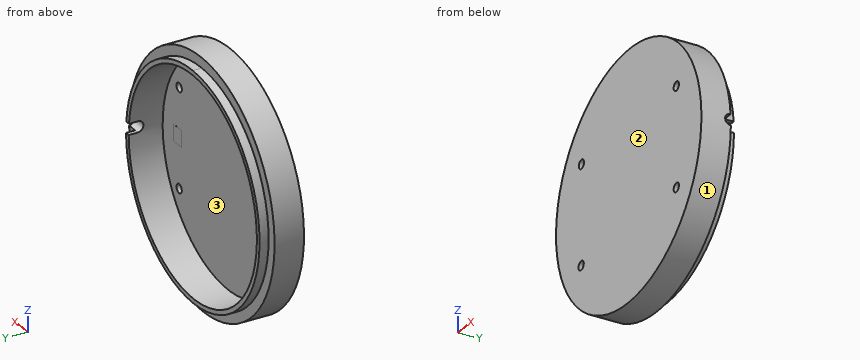
```python
from build123d import *

# Parameters (mm, degrees)
SKETCH2_R                = 55
BOSS_EXTRUDE2_DEPTH      = 13
SKETCH7_R                = 50.5
BOSS_EXTRUDE3_DEPTH      = 4
SKETCH8_R                = 48.5
CUT_EXTRUDE3_DEPTH       = 15
SKETCH9_R                = 2
SKETCH9_W                = 3.162660916
SKETCH9_H                = 2.60493009
CUT_EXTRUDE4_DEPTH       = 15
CUT_EXTRUDE5_DEPTH       = 20
CUT_EXTRUDE5_DEPTH_BACK  = 1
SKETCH10_R               = 2.5
BOSS_EXTRUDE5_DEPTH      = 0.01
BOSS_EXTRUDE5_DEPTH_BACK = 2
SKETCH11_W               = 6.274273212
SKETCH11_H               = 7.379534018
CUT_EXTRUDE6_REACH       = 81.618
CUT_EXTRUDE6_END_RADIUS  = 50.5
SKETCH13_W               = 5
SKETCH13_H               = 6.11505402


with BuildPart() as part:
    # Sketch2 → Boss-Extrude2 (new body)
    with BuildSketch(Plane(origin=(0, 0, 0), x_dir=(1, 0, 0), z_dir=(0, 1, 0))):
        with Locations(Location((0, 0, 0), (0, 0, 90))):
            Circle(SKETCH2_R)
    extrude(amount=BOSS_EXTRUDE2_DEPTH)

    # Sketch7 → Boss-Extrude3 (add)
    with BuildSketch(Plane(origin=(0, 13, 0), x_dir=(1, 0, 0), z_dir=(0, 1, 0))):
        with Locations(Location((0, 0, 0), (0, 0, 270))):
            Circle(SKETCH7_R)
    extrude(amount=BOSS_EXTRUDE3_DEPTH)

    # Sketch8 → Cut-Extrude3 (cut)
    with BuildSketch(Plane(origin=(0, 17, 0), x_dir=(1, 0, 0), z_dir=(0, 1, 0))):
        with Locations(Location((0, 0, 0), (0, 0, 270))):
            Circle(SKETCH8_R)
    extrude(amount=-CUT_EXTRUDE3_DEPTH, mode=Mode.SUBTRACT)

    # Sketch9 → Cut-Extrude4 (cut)
    with BuildSketch(Plane(origin=(0, 2, 0), x_dir=(1, 0, 0), z_dir=(0, 1, 0))):
        with Locations(Location((36, -22, 0), (0, 0, 270))):
            Circle(SKETCH9_R)
        with Locations(Location((-36, 22, 0), (0, 0, 270))):
            Circle(SKETCH9_R)
        with Locations(Location((-35.8, -22, 0), (0, 0, 270))):
            Circle(SKETCH9_R)
        with Locations(Location((36, 22, 0), (0, 0, 270))):
            Circle(SKETCH9_R)
        with Locations((37.581330458, -0.802465045)):
            Rectangle(SKETCH9_W, SKETCH9_H)
    extrude(amount=-CUT_EXTRUDE4_DEPTH, mode=Mode.SUBTRACT)

    # Sketch10 → Cut-Extrude5 (cut, two sides: drawn at the far end of the back side and taken through both)
    with BuildSketch(Plane(origin=(36, 0, 0), x_dir=(0, 0, -1), z_dir=(1, 0, 0)).offset(-CUT_EXTRUDE5_DEPTH_BACK)):
        with Locations(Location((-2, 13, 0), (0, 0, 180))):
            Circle(SKETCH10_R)
    extrude(amount=CUT_EXTRUDE5_DEPTH + CUT_EXTRUDE5_DEPTH_BACK, mode=Mode.SUBTRACT)

    # Sketch11 → Boss-Extrude5 (add, two sides: drawn at the far end of the back side and taken through both)
    with BuildSketch(Plane(origin=(0, 2, 0), x_dir=(1, 0, 0), z_dir=(0, 1, 0)).offset(-BOSS_EXTRUDE5_DEPTH_BACK)):
        with Locations((37.193701051, -0.388212482)):
            Rectangle(SKETCH11_W, SKETCH11_H)
    extrude(amount=BOSS_EXTRUDE5_DEPTH + BOSS_EXTRUDE5_DEPTH_BACK)

    # Cut-Extrude6: up to this cylinder (the profile starts inside it)
    cut_extrude6_end = Plane(origin=(0, 16.057527, 0), z_dir=(0, -1, 0)) * Cylinder(CUT_EXTRUDE6_END_RADIUS, 265.236, mode=Mode.PRIVATE)
    # Sketch13 → Cut-Extrude6 (cut, up to the surface)
    with BuildSketch(Plane(origin=(0, 0, 0), x_dir=(0, 0, -1), z_dir=(1, 0, 0)), mode=Mode.PRIVATE) as cut_extrude6_sk1:
        with Locations((-2, 16.05752701)):
            Rectangle(SKETCH13_W, SKETCH13_H)
    cut_extrude6_tool1 = extrude(cut_extrude6_sk1.sketch, amount=CUT_EXTRUDE6_REACH, mode=Mode.PRIVATE) & cut_extrude6_end
    add(cut_extrude6_tool1.solids().sort_by_distance((0, 16.057527, 2))[0], mode=Mode.SUBTRACT)


solid = part.part
```
Input: part model. Units: mm. Frame: model coordinates. Face numbers are marked on the shaded views. Round coordinates to 2 decimals unless told otherwise and drop trailing zeros. Loops run counter-clockwise (first coordinate to the right, second up) from the corner with the lowest first, then second, coordinate; pieces in that order, holes last. Notation, with made-up numbers: (48.25, 21.25) -> (57.25, 21.25) arc R27 ccw to (57.25, 43.25) -> close; hole circle Ø4 at (6.25, -10). An arc over 180 degrees is marked (long way). Write each question's results on one line, items separated by ' | '.
1. Section B-B (x = 14.5). Return loops of the section in (y, z).
Geometry results:
outline: (0, -53.05) -> (13, -53.05) -> (13, -48.37) -> (17, -48.37) -> (17, -46.28) -> (2, -46.28) -> (2, 46.28) -> (17, 46.28) -> (17, 48.37) -> (13, 48.37) -> (13, 53.05) -> (0, 53.05) -> close
2. First-contact query: P1, Ø10, axis at y = 3.5, z = 24.5, coming from the +X side; P2, Ø5, axis at x = -41.5, y = 13, coming from the +Z side; P3, Ø10, axis at y = 2.5, z = 14.5, coming from the -X side. Flat tips, straight axial feed; report the tip coordinate or a pass-through.
Geometry results:
P1: x = 51.43 | P2: z = 38.78 | P3: x = -54.17
3. Section A-A (z = 22). Return loops of the section in (x, y).
Geometry results:
outline: (-50.41, 0) -> (-37.8, 0) -> (-37.8, 2) -> (-43.22, 2) -> (-43.22, 17) -> (-45.46, 17) -> (-45.46, 13) -> (-50.41, 13) -> close; (-33.8, 0) -> (34, 0) -> (34, 2) -> (-33.8, 2) -> close; (38, 0) -> (50.41, 0) -> (50.41, 13) -> (45.46, 13) -> (45.46, 17) -> (43.22, 17) -> (43.22, 2) -> (38, 2) -> close
4. Ray query, line 1 (X direction, y = 9.5, z = 0); line 2 (X direction, y = 0.45, z = 22); line 3 (X direction, y = 0.5, z = -22). Return the intervals inside material, ascending. Write a range as from..to.
Geometry results:
line 1: -55..-48.5, 48.5..55 | line 2: -50.41..-37.8, -33.8..34, 38..50.41 | line 3: -50.41..-38, -34..34, 38..50.41
5. Section C-C (y = 4.5). Return loops of the section in (x, z).
Geometry results:
outline: circle Ø110 at (0, 0); hole circle Ø97 at (0, 0)
6. Mould query, pull axis X, two halves, no side actions, for the marked faces 1, 2 and 3. Classes: +X half, -X half, draft (parallel to the pull), parting line (faces both ways), or undercut.
Geometry results:
face 1: parting line | face 2: draft | face 3: undercut
7. Section D-D (z = 6.5). Return loops of the section in (x, y).
Geometry results:
outline: (-54.61, 0) -> (54.61, 0) -> (54.61, 13) -> (50.08, 13) -> (50.08, 17) -> (48.06, 17) -> (48.06, 2) -> (-48.06, 2) -> (-48.06, 17) -> (-50.08, 17) -> (-50.08, 13) -> (-54.61, 13) -> close
